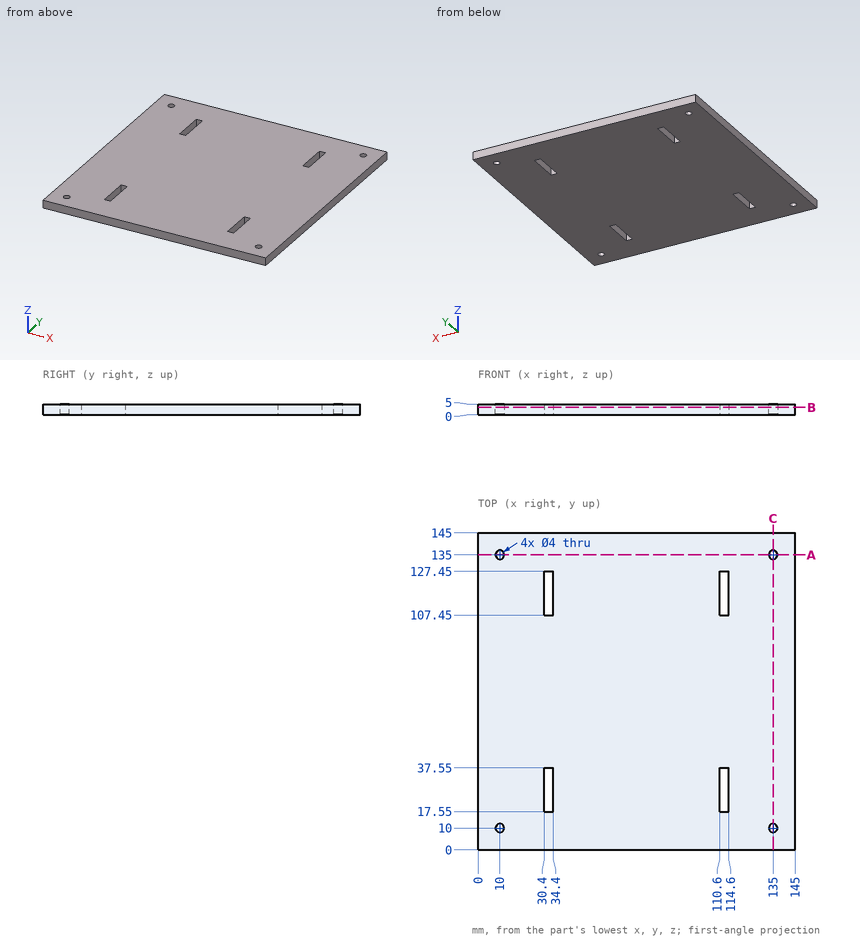
Study the drawing (mm; zero at the part's minimum x, y, z) and answer. Coordinates: 2 decimals unless noted, no trailing zeros. Loops run counter-clockwise (first coordinate to the right, second up) from the corner with the lowest first, then second, coordinate; pieces in that order, holes last. Notation, with made-up numbers: (44, 29) -> (83, 29) arc R15 cw to (83, 35) -> close; hole circle Ø5 at (26, 64.5). An arc over 180 degrees is marked (long way). Write item = value, one per line. Start each with the question number.
1) Find the intervals of material crossed by L1, parallel to Y at x = 135, z = 2; L2, parallel to X at y = 117, z = 0.5, in increasing order. Write a range as from..to.
2) The part is cut by section B-B, the plane z = 3.4. State how many separate pieces and enclosed holes the cut face has, plus the area to 3 significant figures.
3) The part is cut by section A-A, the plane y = 135. Determine the outline of the cut face in (x, z).
Result:
q1.L1 = 0..8, 12..133, 137..145
q1.L2 = 0..30.4, 34.4..110.6, 114.6..145
q2.separate_pieces = 1
q2.enclosed_holes = 8
q2.area = 20,700 mm²
q3.outline = (0, 0) -> (8, 0) -> (8, 5) -> (0, 5) -> close; (12, 0) -> (133, 0) -> (133, 5) -> (12, 5) -> close; (137, 0) -> (145, 0) -> (145, 5) -> (137, 5) -> close
